For this review, take the finished solid that the model builds, in its own axes (mm). A direction names the side the tool comes from. Give positions to 0.01 mm unless a question says otherwise; leave off trailing zeros. Order: outer loops, then holes, each group sorted by start corner. A loop starts at its lowest first (then second) coordinate and runs counter-clockwise, first axis right, second up. Notation, with made-up numbers: (48, 22) -> (89, 22) arc R21 ccw to (89, 55) -> close; hole circle Ø7 at (22.5, 76.25). An arc over 180 degrees is marked (long way). Return JSON: item names as keys, results as strings. Group by question number.
1) Add section B-B (y = 0). Give the boundary of the cut face in (x, z).
2) Add section C-C (x = 11.5). Give the boundary of the cut face in (y, z), then the cut area to 3 significant figures.
3) Insertion check: P1, Ø5, axis at x = -9, y = -11, coming from the +Z side; P2, Ø2.5, axis at x = 0, y = 12.5, coming from the +Z side; P3, Ø7, axis at x = -1.5, y = -1.5, coming from the -Z side; P4, Ø4, axis at y = 5.5, z = 9.5, coming from the -X side. Each pin has a flat end and moves straight along its axis. Give the tip position at first contact, or say it passes through.
4) The part is to be moulded in two halves that separate along X. For faces 4 (the face through (-13.887, 10.648, 1.479)), 5 (the face through (4, -4, 14)), 6 (the face through (0.65, 10.93, 1.99)), say which applies: released by +X, released by -X, zero draft, split by the parting line, or undercut.
5) For faces 1 (the face through (12.485, -5.881, 1.986)), 2 (the face through (-1.172, -8.923, 8.423)), 3 (the face through (-2, -5, 1)), list the 3-axis set-ups (+Z, -Z, +X, -X, +Y, -Y) from which the entire face can be reached by the end or side of a thin tool; tool diameter is ignored.
6) Add section D-D (y = -6.25). Give the boundary of the cut face in (x, z), then the cut area to 3 significant figures.
7) To check wall thickness, follow line 1 along Y through (x, z) = (0, 1.95); line 2 along Y through (x, z) = (0, 0.4); line 3 along X through (y, z) = (-6.25, 2.25). State the ranges of each line that lie inside material, in increasing order.
8) Add section A-A (x = 0). Give the boundary of the cut face in (y, z), then the cut area to 3 significant figures.
Autodesk Inventor part; units mm, degrees
ref_plane "YZ Plane" through (0, 0, 0) normal (1, 0, 0) x (0, 1, 0)
ref_plane "XZ Plane" through (0, 0, 0) normal (0, 1, 0) x (-1, 0, 0)
ref_plane "XY Plane" through (0, 0, 0) normal (0, 0, 1) x (1, 0, 0)
sketch "スケッチ1" plane through (0, 0, 0) normal (0, 0, 1) x (1, 0, 0)
  circle A0 centre (0, 0) radius 17.5
  dimension "d0" = 35
extrude "押し出し1" add sketch "スケッチ1" along normal blind 3
sketch "スケッチ2" plane through (0, 0, 3) normal (0, 0, 1) x (1, 0, 0)
  circle A0 centre (0, 0) radius 9
  dimension "d3" = 18
extrude "押し出し2" add sketch "スケッチ2" along normal blind 11
sketch "スケッチ3" plane through (0, 0, 14) normal (0, 0, 1) x (1, 0, 0)
  point P0 (0, 0)
  point P1 (0, 0)
hole "穴1" at (0, 0, 14) direction (0, 0, -1) diameter 10.106 end through all
sketch "スケッチ5" plane through (0, 0, 0) normal (0, 0, -1) x (-1, 0, 0)
  circle A0 centre (0, 0) radius 7
  dimension "d25" = 14
extrude "押し出し3" cut sketch "スケッチ5" against normal blind 1
sketch "スケッチ8" plane through (0, 0, 3) normal (0, 0, 1) x (1, 0, 0)
  point P0 (0, 0)
  point P1 (0, 12.5)
  point P2 (-10.8253, -6.25)
  point P3 (10.8253, -6.25)
  dimension "d47" = 12.5
  dimension "d50" = 360
hole "穴4" at (0, 12.5, 3) at (-10.8253, -6.25, 3) at (10.8253, -6.25, 3) direction (0, 0, -1) diameter 3.4 end through all
sketch "スケッチ9" plane through (0, 0, 0) normal (0, 0, -1) x (-1, 0, 0)
  circle A0 centre (0, 12.5) radius 3
  circle A1 centre (-10.8253, -6.25) radius 3
  circle A2 centre (10.8253, -6.25) radius 3
  point P0 (0, 0)
  dimension "d59" = 6
  dimension "d60" = 12.5
  dimension "d63" = 360
extrude "押し出し5" cut sketch "スケッチ9" against normal blind 1
properties part number "製図規定課題2"
Evaluation:
{
 "1": {"outline": "(-17.5, 0) -> (-7, 0) -> (-7, 1) -> (-5.05, 1) -> (-5.05, 14) -> (-9, 14) -> (-9, 3) -> (-17.5, 3) -> close; (5.05, 1) -> (7, 1) -> (7, 0) -> (17.5, 0) -> (17.5, 3) -> (9, 3) -> (9, 14) -> (5.05, 14) -> close"},
 "2": {"outline": "(-13.19, 0) -> (-9.17, 0) -> (-9.17, 1) -> (-7.81, 1) -> (-7.81, 3) -> (-13.19, 3) -> close; (-4.69, 1) -> (-3.33, 1) -> (-3.33, 0) -> (13.19, 0) -> (13.19, 3) -> (-4.69, 3) -> close", "area": "67.1 mm^2"},
 "3": {"P1": "z = 3", "P2": "through", "P3": "z = 1", "P4": "x = -8.29"},
 "4": {"face 4": "split by the parting line", "face 5": "zero draft", "face 6": "undercut"},
 "5": {"face 1": "+Z, -Z", "face 2": "+Z", "face 3": "-Z"},
 "6": {"outline": "(-16.35, 0) -> (-13.83, 0) -> (-13.83, 1) -> (-12.53, 1) -> (-12.53, 3) -> (-16.35, 3) -> close; (-9.13, 1) -> (-7.83, 1) -> (-7.83, 0) -> (-3.15, 0) -> (-3.15, 1) -> (3.15, 1) -> (3.15, 0) -> (7.83, 0) -> (7.83, 1) -> (9.13, 1) -> (9.13, 3) -> (6.48, 3) -> (6.48, 14) -> (-6.48, 14) -> (-6.48, 3) -> (-9.13, 3) -> close; (12.53, 1) -> (13.83, 1) -> (13.83, 0) -> (16.35, 0) -> (16.35, 3) -> (12.53, 3) -> close", "area": "209 mm^2"},
 "7": {"line 1": "-17.5 to -5.05, 5.05 to 10.8, 14.2 to 17.5", "line 2": "-17.5 to -7, 7 to 9.5, 15.5 to 17.5", "line 3": "-16.35 to -12.53, -9.13 to 9.13, 12.53 to 16.35"},
 "8": {"outline": "(-17.5, 0) -> (-7, 0) -> (-7, 1) -> (-5.05, 1) -> (-5.05, 14) -> (-9, 14) -> (-9, 3) -> (-17.5, 3) -> close; (5.05, 1) -> (7, 1) -> (7, 0) -> (9.5, 0) -> (9.5, 1) -> (10.8, 1) -> (10.8, 3) -> (9, 3) -> (9, 14) -> (5.05, 14) -> close; (14.2, 1) -> (15.5, 1) -> (15.5, 0) -> (17.5, 0) -> (17.5, 3) -> (14.2, 3) -> close", "area": "145 mm^2"}
}
